Work out the finished part from the listing and answer in its coordinate system (mm). Face numbers are marked on the shaded views. A direction names the side the tool comes from. Give positions to 0.01 mm unless a question says otherwise; leave off trailing zeros. Loops run counter-clockwise (first coordinate to the right, second up) from the corner with the lowest first, then second, coordinate; pieces in that order, holes last. Notation, with made-up numbers: (67.5, -39.5) - (126.5, -39.5) arc R16 ccw to (126.5, -22.5) - close; hole circle Ø7 at (53.25, -23). An arc over 180 degrees is marked (long way). Use CSV: the item, a comma, the result in double quotes.
from build123d import *

# Parameters (mm, degrees)
CROQUIS1_W                       = 60
CROQUIS1_H                       = 80
BRIDA_BASE1_DEPTH                = 5
BRIDA_DE_ARISTA1_STRIP_W         = 21.4732
BRIDA_DE_ARISTA1_STRIP_H         = 5
BRIDA_DE_ARISTA1_STRIP_CUT_DEPTH = 80
BRIDA_DE_ARISTA1_DEPTH           = 80
CROQUIS9_R                       = 2.5
CORTAR_EXTRUIR1_DEPTH            = 5


# Sheet-metal steps are written as plain solids
with BuildPart() as part:
    # Croquis1 → Brida base1 (new body)
    with BuildSketch(Plane(origin=(0, 0, 0), x_dir=(1, 0, 0), z_dir=(0, 1, 0))):
        Rectangle(CROQUIS1_W, CROQUIS1_H)
    extrude(amount=-BRIDA_BASE1_DEPTH)

    # Brida de arista1 strip (across the edge) → Brida de arista1 strip cut (cut)
    with BuildSketch(Plane(origin=(30, 0, 40), x_dir=(-1, 0, 0), z_dir=(0, 0, -1))):
        with Locations((-5, -2.5)):
            Rectangle(BRIDA_DE_ARISTA1_STRIP_W, BRIDA_DE_ARISTA1_STRIP_H)
    extrude(amount=BRIDA_DE_ARISTA1_STRIP_CUT_DEPTH, mode=Mode.SUBTRACT)

    # Brida de arista1 section (across the edge) → Brida de arista1 (add)
    with BuildSketch(Plane(origin=(30, 0, 40), x_dir=(-1, 0, 0), z_dir=(0, 0, -1))):
        with BuildLine():
            Line((0, 0.7366), (0, 16))
            Line((0, 16), (5, 16))
            Line((5, 16), (5, 0.7366))
            ThreePointArc((5, 0.7366), (5.215745145, 0.215745145), (5.7366, 0))
            Line((5.7366, 0), (5.7366, -5))
            ThreePointArc((5.7366, -5), (1.680211239, -3.319788761), (0, 0.7366))
        make_face()
    extrude(amount=BRIDA_DE_ARISTA1_DEPTH)

    # Croquis9 → Cortar-Extruir1 (cut)
    with BuildSketch(Plane(origin=(0, 0, 0), x_dir=(1, 0, 0), z_dir=(0, 1, 0))):
        with Locations(Location((-13.75, 30.13, 0), (0, 0, 270))):
            Circle(CROQUIS9_R)
        with Locations(Location((13.75, 30.13, 0), (0, 0, 270))):
            Circle(CROQUIS9_R)
        with Locations(Location((13.75, -30.12, 0), (0, 0, 270))):
            Circle(CROQUIS9_R)
        with Locations(Location((-13.75, -30.12, 0), (0, 0, 270))):
            Circle(CROQUIS9_R)
    extrude(amount=-CORTAR_EXTRUIR1_DEPTH, mode=Mode.SUBTRACT)


solid = part.part
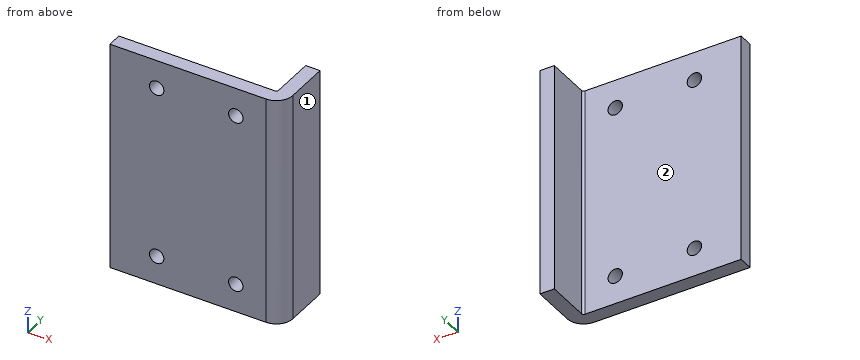
Item 1: A cutting plane is placed at A-A on z = 30.12. Determine the outline of the cut face in (x, y).
Determined:
outline,"(-30, -5) - (-16.25, -5) - (-16.25, 0) - (-30, 0) - close; (-11.25, -5) - (11.25, -5) - (11.25, 0) - (-11.25, 0) - close; (16.25, -5) - (24.26, -5) arc R5.74 ccw to (30, 0.74) - (30, 16) - (25, 16) - (25, 0.74) arc R0.74 cw to (24.26, 0) - (16.25, 0) - close"
Item 2: A cutting plane is placed at B-B on x = 13.75. Determine the outline of the cut face in (y, z).
Determined:
outline,"(-5, -40) - (0, -40) - (0, -32.63) - (-5, -32.63) - close; (-5, -27.63) - (0, -27.63) - (0, 27.62) - (-5, 27.62) - close; (-5, 32.62) - (0, 32.62) - (0, 40) - (-5, 40) - close"
Item 3: For the marked faces 1 and 2, determine the directions among +Z, -Z, +X, -X, +Y, -Y from which every point of the face is accessible in a straight line to the end or side of a thin tool.
Determined:
face 1,"+Z, -Z, +X, +Y, -Y"
face 2,"+Z, -Z, -X, +Y"
Item 4: A cutting plane is placed at C-C on z = 22. Determine the outline of the cut face in (x, y), and give its area (3 significant figures).
Determined:
outline,"(-30, -5) - (24.26, -5) arc R5.74 ccw to (30, 0.74) - (30, 16) - (25, 16) - (25, 0.74) arc R0.74 cw to (24.26, 0) - (-30, 0) - close"
area,"373 mm²"
Item 5: A cutting plane is placed at D-D on y = -1.5. Determine the outline of the cut face in (x, z), and give its area (3 significant figures).
Determined:
outline,"(-30, -40) - (29.55, -40) - (29.55, 40) - (-30, 40) - close; hole circle Ø5 at (-13.75, -30.13); hole circle Ø5 at (-13.75, 30.12); hole circle Ø5 at (13.75, -30.13); hole circle Ø5 at (13.75, 30.12)"
area,"4,690 mm²"
Item 6: Given P1, Ø7.5, axis at y = 8.5, z = -8, coming from the -X side; P2, Ø8, axis at x = 2, z = -29, coming from the +Y side; P3, Ø1, axis at y = -2, z = -7.5, coming from the +X side; P4, Ø3, axis at x = 13.75, z = 30.12, coming from the -Y side, each flat-ended and moving along its own axis, determine where each tip first touches the part or whether it passes through.
Determined:
P1,"stops at x = 25"
P2,"stops at y = 0"
P3,"stops at x = 29.55"
P4,"passes through"
Item 7: Find the intervals of material crossed by line 1 (X direction, y = -2.9, z = -30.13); line 2 (X direction, y = -3.1, z = -30.13); line 3 (Z direction, x = -15, y = -2.5), in increasing order.
Determined:
line 1,"x = -30 to -16.25, -11.25 to 11.25, 16.25 to 28.7"
line 2,"x = -30 to -16.25, -11.25 to 11.25, 16.25 to 28.53"
line 3,"z = -40 to -32.3, -27.96 to 27.95, 32.29 to 40"
